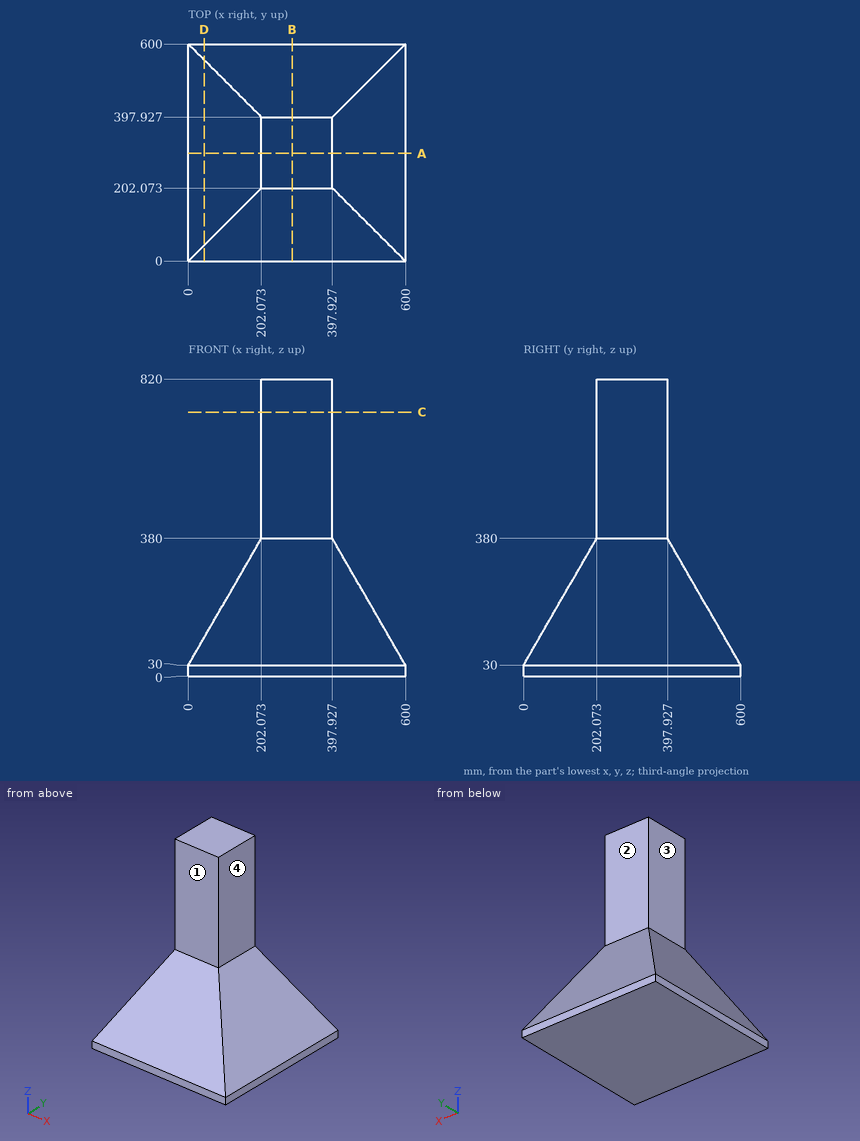
Can you work these out from the drawing? Everything is in mm from the part's minimum corner. A direction names the side the tool comes from. Coordinates: 2 decimals unless noted, no trailing zeros. Loops run counter-clockwise (first coordinate to the right, second up) from the corner with the lowest first, then second, coordinate; pieces in that order, holes last. Notation, with made-up numbers: M 60.5,37.25 L 67.5,37.25 A8 cw 67.5,49.25 Z; hole C 5,45 d2. An arc over 180 degrees is marked long. Put each result on its own line as item: value. Start each with the question number.
(1) Will these pins go through, and if not, where does the flat tip stop? P1, Ø12, axis at x = 364, y = 308, coming from the -Z side; P2, Ø10, axis at x = 477, z = 155.5, coming from the +Y side; P3, Ø12, axis at y = 390.5, z = 228.5, coming from the +X side; P4, Ø5, axis at x = 400.5, z = 585.5, coming from the -Y side.
(2) Suppose I cut it at D-D on x = 44. Please give me the cut outline in (y, z), then the cut area to 3 significant figures.
(3) For the marked faces 1, 2, 3 and 4, which set-ups out of +Z, -Z, +X, -X, +Y, -Y let a thin tool reach every point of the face, with its end or its side?
(4) Suppose I cut it at A-A on y = 298. Please give me the cut outline in (x, z).
(5) I need wall thicknesses on line 1 (X direction, y = 329.5, z = 738.5); line 2 (Z direction, x = 478, y = 268.5). Which ranges of each line are inside material? Lowest first, please. Write a range as from..to.
(6) Suppose I cut it at C-C on z = 729. Please give me the cut outline in (x, y).
Solutions:
1. P1: stops at z = 0
1. P2: stops at y = 530.43
1. P3: stops at x = 488.86
1. P4: passes through
2. outline: M 0,0 L 600,0 L 600,30 L 556,106.21 L 44,106.21 L 0,30 Z
2. area: 60,400 mm2
3. face 1: +Z, +X, -X, -Y
3. face 2: +Z, +X, -X, +Y
3. face 3: +Z, -X, +Y, -Y
3. face 4: +Z, +X, +Y, -Y
4. outline: M 0,0 L 600,0 L 600,30 L 397.93,380 L 397.93,820 L 202.07,820 L 202.07,380 L 0,30 Z
5. line 1: x = 202.07..397.93
5. line 2: z = 0..241.31
6. outline: M 202.07,202.07 L 397.93,202.07 L 397.93,397.93 L 202.07,397.93 Z
